Here's the drawing with two shaded views (mm, measured from the low corner). I have some questions. Round coordinates to 2 decimals unless told otherwise and drop trailing zeros. Order: outer loops, then holes, each group sorted by start corner. A loop starts at its lowest first (then second) coordinate and runs counter-clockwise, first axis right, second up. Notation, with made-up numbers: (57, 10.5) -> (103, 10.5) arc R26 ccw to (103, 44.5) -> close; hole circle Ø1 at (37.5, 67.25). An arc over 180 degrees is marked (long way). Answer in a Markdown table with one row per item.
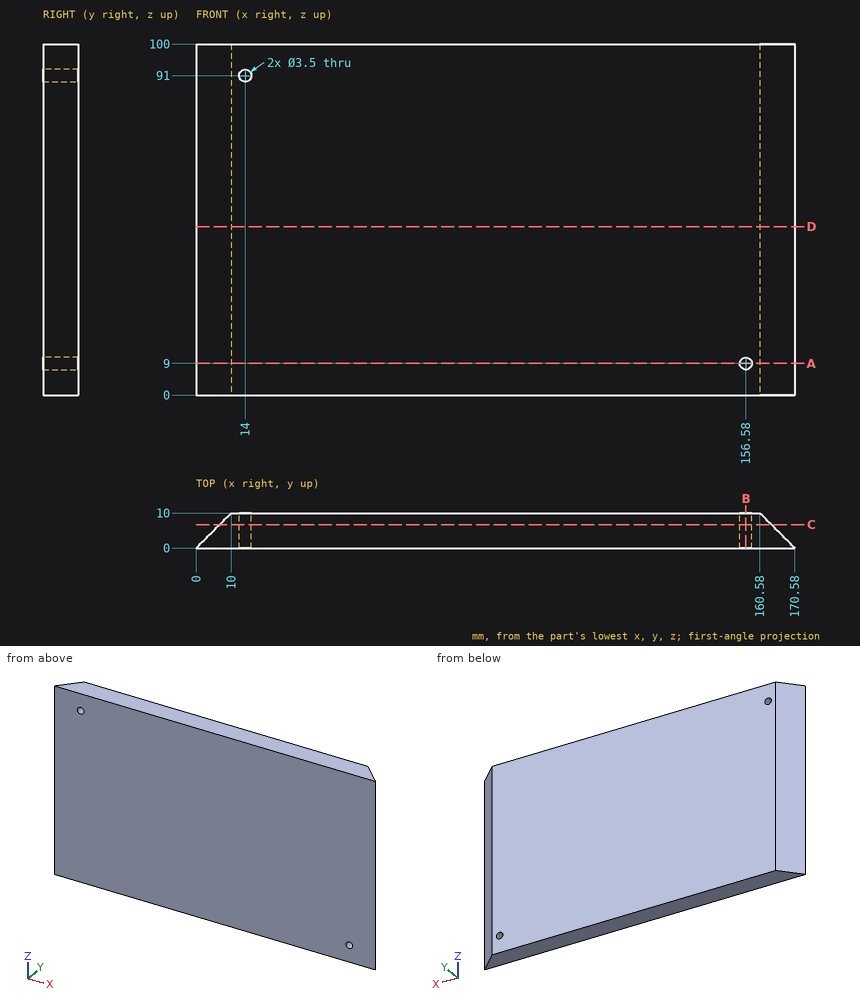
1. Suppose I cut it at C-C on y = 6.75. Write out the boundary of the cut face in (x, z).
Numbers:
| item | result |
|---|---|
| outline | (6.75, 0) -> (163.83, 0) -> (163.83, 100) -> (6.75, 100) -> close; hole circle Ø3.5 at (14, 91); hole circle Ø3.5 at (156.58, 9) |
2. Please list where these lines run through material, in increasing order: line 1 along X through (y, z) = (6.75, 9); line 2 along Z through (x, y) = (156.58, 2.5); line 3 along X through (y, z) = (5.25, 91).
Numbers:
| item | result |
|---|---|
| line 1 | x = 6.75 to 154.83, 158.33 to 163.83 |
| line 2 | z = 0 to 7.25, 10.75 to 100 |
| line 3 | x = 5.25 to 12.25, 15.75 to 165.33 |
3. Suppose I cut it at B-B on x = 156.58. Write out the boundary of the cut face in (y, z).
Numbers:
| item | result |
|---|---|
| outline | (0, 0) -> (10, 0) -> (10, 7.25) -> (0, 7.25) -> close; (0, 10.75) -> (10, 10.75) -> (10, 100) -> (0, 100) -> close |
4. Suppose I cut it at D-D on z = 48. Write out the boundary of the cut face in (x, y).
Numbers:
| item | result |
|---|---|
| outline | (0, 0) -> (170.58, 0) -> (160.58, 10) -> (10, 10) -> close |
5. Suppose I cut it at A-A on z = 9. Write out the boundary of the cut face in (x, y), then the cut area to 3 significant figures.
Numbers:
| item | result |
|---|---|
| outline | (0, 0) -> (154.83, 0) -> (154.83, 10) -> (10, 10) -> close; (158.33, 0) -> (170.58, 0) -> (160.58, 10) -> (158.33, 10) -> close |
| area | 1,570 mm2 |
6. For pin 1 Ø5 at (y, z) = (5.5, 57.5) entering from -X; pin 2 Ø1.5 at (y, z) = (7, 42.5) entering from -X; pin 3 Ø6 at (y, z) = (3.5, 56.5) entering from +X, each with a flat end and sliding along its axis, tell me the tip position at first contact or that it passes through.
Numbers:
| item | result |
|---|---|
| pin 1 | stops at x = 3 |
| pin 2 | stops at x = 6.25 |
| pin 3 | stops at x = 170.08 |
